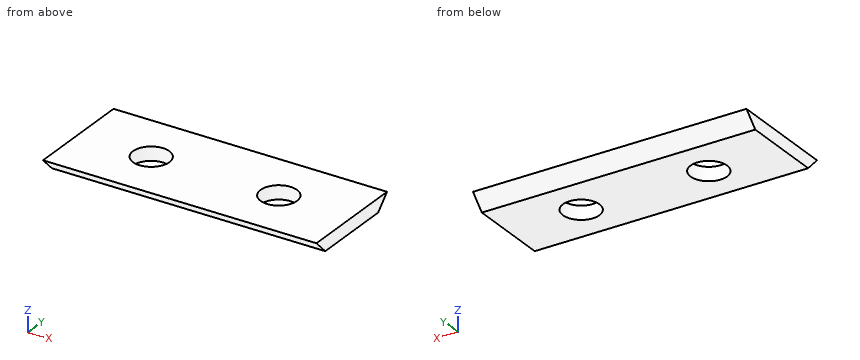
from build123d import *

# Parameters (mm, degrees)
SKETCH1_W           = 30
SKETCH1_H           = 12
SKETCH1_R           = 2
BOSS_EXTRUDE1_DEPTH = 1.5
CUT_EXTRUDE1_DEPTH  = 31


with BuildPart() as part:
    # Sketch1 → Boss-Extrude1 (new body)
    with BuildSketch(Plane.XY):
        with Locations((-15, 6)):
            Rectangle(SKETCH1_W, SKETCH1_H)
        with Locations((-22, 6)):
            Circle(SKETCH1_R, mode=Mode.SUBTRACT)
        with Locations((-8, 6)):
            Circle(SKETCH1_R, mode=Mode.SUBTRACT)
    extrude(amount=BOSS_EXTRUDE1_DEPTH)

    # Sketch2 → Cut-Extrude1 (cut, through all)
    with BuildSketch(Plane(origin=(0, 0, 0), x_dir=(0, 0, -1), z_dir=(1, 0, 0))):
        Polygon((0, 12), (-1.5, 12), (0, 10.5), align=None)
        Polygon((0, 0), (0, 1.5), (-1.5, 0), align=None)
    extrude(amount=-CUT_EXTRUDE1_DEPTH, mode=Mode.SUBTRACT)


solid = part.part
Check sheet for the modelled part. Datum: model origin and axes. Units: mm. Round coordinates to 2 decimals unless told otherwise and drop trailing zeros. Order: outer loops, then holes, each group sorted by start corner. A loop starts at its lowest first (then second) coordinate and runs counter-clockwise, first axis right, second up.
Q1. Cross-section at B-B, the plane y = 6. Enter the section's corners in (x, z), plus the area to 3 significant figures.
Filled sheet:
outline: (-30, 0) - (-24, 0) - (-24, 1.5) - (-30, 1.5) - close; (-20, 0) - (-10, 0) - (-10, 1.5) - (-20, 1.5) - close; (-6, 0) - (0, 0) - (0, 1.5) - (-6, 1.5) - close
area: 33.0 mm2
Q2. Cross-section at D-D, the plane x = -9. Enter the section's corners in (y, z), plus the area to 3 significant figures.
Filled sheet:
outline: (0, 1.5) - (1.5, 0) - (4.27, 0) - (4.27, 1.5) - close; (7.73, 0) - (10.5, 0) - (12, 1.5) - (7.73, 1.5) - close
area: 10.6 mm2
Q3. Cross-section at C-C, the plane z = 0.9. Enter the section's corners in (x, y).
Filled sheet:
outline: (-30, 0.6) - (0, 0.6) - (0, 11.4) - (-30, 11.4) - close; hole circle Ø4 at (-22, 6); hole circle Ø4 at (-8, 6)
Q4. Cross-section at A-A, the plane x = -22. Enter the section's corners in (y, z), plus the area to 3 significant figures.
Filled sheet:
outline: (0, 1.5) - (1.5, 0) - (4, 0) - (4, 1.5) - close; (8, 0) - (10.5, 0) - (12, 1.5) - (8, 1.5) - close
area: 9.75 mm2
Q5. Scan lines: L1, parallel to X at y = 7.75, z = 0.2; L2, parallel to X at y = 4.75, z = 0.25; L3, parallel to Y at x = -8, z = 0.45. Record each from-to range of solid material in increasing order.
Filled sheet:
L1: x = -30 to -22.97, -21.03 to -8.97, -7.03 to 0
L2: x = -30 to -23.56, -20.44 to -9.56, -6.44 to 0
L3: y = 1.05 to 4, 8 to 10.95
